```python
from build123d import *

# Parameters (mm, degrees)
SKETCH1_R           = 1.5
BOSS_EXTRUDE1_DEPTH = 1.6


with BuildPart() as part:
    # Sketch1 → Boss-Extrude1 (new body)
    with BuildSketch(Plane.XY):
        with BuildLine():
            Line((-9.5, -12.5), (9.5, -12.5))
            ThreePointArc((9.5, -12.5), (11.621320344, -11.621320344), (12.5, -9.5))
            Line((12.5, -9.5), (12.5, 9.5))
            ThreePointArc((12.5, 9.5), (11.621320344, 11.621320344), (9.5, 12.5))
            Line((9.5, 12.5), (-9.5, 12.5))
            ThreePointArc((-9.5, 12.5), (-11.621320344, 11.621320344), (-12.5, 9.5))
            Line((-12.5, 9.5), (-12.5, -9.5))
            ThreePointArc((-12.5, -9.5), (-11.621320344, -11.621320344), (-9.5, -12.5))
        make_face()
        with Locations((-10, 10)):
            Circle(SKETCH1_R, mode=Mode.SUBTRACT)
        with Locations(Location((10, 10, 0), (0, 0, 180))):
            Circle(SKETCH1_R, mode=Mode.SUBTRACT)
        with Locations((10, -10)):
            Circle(SKETCH1_R, mode=Mode.SUBTRACT)
        with Locations(Location((-10, -10, 0), (0, 0, 180))):
            Circle(SKETCH1_R, mode=Mode.SUBTRACT)
    extrude(amount=BOSS_EXTRUDE1_DEPTH)


solid = part.part
```
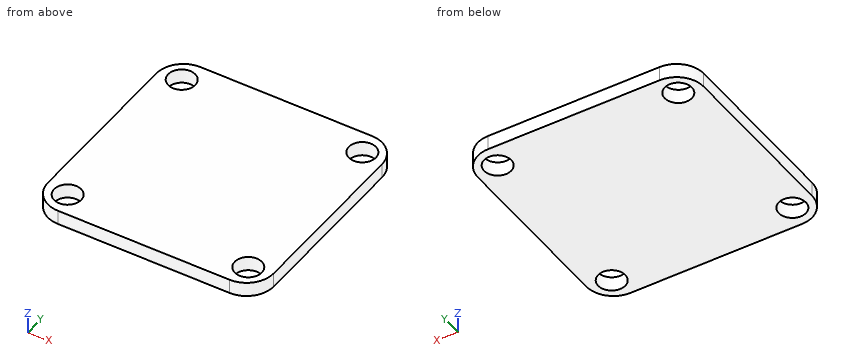
The listing builds one solid part. Answer for the finished solid, in the listing's coordinates (mm). Coordinates: 2 decimals unless noted, no trailing zeros. Write each loop counter-clockwise with the first axis right and the second up, starting at its lowest first coordinate (ties: lowest second). Pieces come first, ordered by that corner, then holes. Notation, with made-up numbers: (34, 29.5) - (71, 29.5) arc R9 ccw to (71, 35.5) - close; hole circle Ø9 at (73.25, 69). An arc over 180 degrees is marked (long way). Return JSON: item names as keys, results as strings. Group by question number.
1. A cutting plane is placed at B-B, the plane z = 1.2. Determine the outline of the cut face in (x, y).
2. A cutting plane is placed at A-A, the plane x = -10. Determine the outline of the cut face in (y, z).
3. Straight lines are drawn through the part: L1, parallel to Y at x = 10, z = 1.35; L2, parallel to Y at x = -11, z = 0.8; L3, parallel to X at y = -10.5, z = 0.8. For each, find the intervals that lie inside material, in ascending order.
4. Given pin 1 (2.5 mm diameter, centred on x = -10, y = 10, fed in from +Z), flat-ended and moving along its own axis, determine where the tip first touches the part or whether it passes through.
Ans:
{
 "1": {"outline": "(-12.5, -9.5) arc R3 ccw to (-9.5, -12.5) - (9.5, -12.5) arc R3 ccw to (12.5, -9.5) - (12.5, 9.5) arc R3 ccw to (9.5, 12.5) - (-9.5, 12.5) arc R3 ccw to (-12.5, 9.5) - close; hole circle Ø3 at (-10, -10); hole circle Ø3 at (-10, 10); hole circle Ø3 at (10, -10); hole circle Ø3 at (10, 10)"},
 "2": {"outline": "(-12.46, 0) - (-11.5, 0) - (-11.5, 1.6) - (-12.46, 1.6) - close; (-8.5, 0) - (8.5, 0) - (8.5, 1.6) - (-8.5, 1.6) - close; (11.5, 0) - (12.46, 0) - (12.46, 1.6) - (11.5, 1.6) - close"},
 "3": {"L1": "-12.46 to -11.5, -8.5 to 8.5, 11.5 to 12.46", "L2": "-12.1 to -11.12, -8.88 to 8.88, 11.12 to 12.1", "L3": "-12.33 to -11.41, -8.59 to 8.59, 11.41 to 12.33"},
 "4": {"pin 1": "through"}
}
